Source: CAD feature listing. Evaluate the final solid. Frame: model axes, mm. A direction names the side the tool comes from. Give positions to 0.01 mm unless a question says otherwise; leave off trailing zeros. Write each loop counter-clockwise with the first axis right and the second up, starting at its lowest first coordinate (ties: lowest second). Pieces come first, ordered by that corner, then holes. Notation, with made-up numbers: M 71,87.5 L 120,87.5 A18 cw 120,95.5 Z; hole C 62.25,3 d9. An arc over 180 degrees is marked long. Use CSV: the item, a comma, the result in double quotes. Start each with the question number.
from build123d import *

# Parameters (mm, degrees)
F1_DEPTH = 240
F2_T     = -15
F3_R     = 50
F4_DEPTH = 50
F5_R     = 75
F6_DEPTH = 50


with BuildPart() as f1:
    # F0 (on Top) → F1 (new body)
    with BuildSketch(Plane.XY):
        with BuildLine():
            Line((0, 420), (0, 0))
            Line((0, 0), (300, 0))
            Line((300, 0), (300, 120))
            Line((300, 120), (220, 120))
            Line((220, 120), (220, 320))
            ThreePointArc((220, 320), (187.6502089709, 540.8304597359), (0, 420))
        make_face()
    extrude(amount=F1_DEPTH)

    # F2
    f2_openings = [f1.faces().sort_by_distance(p)[0] for p in [
        (150, 0, 120),
    ]]
    offset(amount=F2_T, openings=f2_openings, kind=Kind.INTERSECTION)

    # F3 (on face) → F4 (cut)
    with BuildSketch(Plane.XY.offset(240)):
        with Locations((132.7272727273, 420)):
            Circle(F3_R)
    extrude(amount=-F4_DEPTH, mode=Mode.SUBTRACT)

    # F5 (on face) → F6 (cut)
    with BuildSketch(Plane(origin=(0, 0, 0), x_dir=(0, -1, 0), z_dir=(-1, 0, 0))):
        with Locations((-320, 120)):
            Circle(F5_R)
        with Locations((-120, 120)):
            Circle(F5_R)
    extrude(amount=-F6_DEPTH, mode=Mode.SUBTRACT)


solid = f1.part
1. Access query for faces 5 (the cylindrical face through (7.395, 248.463, 142.528)), 6 (the cylindrical face through (126.218, 469.575, 232.605)), 7 (the flat face through (261, 120, 118)), 8 (the flat face through (0, 213, 118)), 9 (the flat face through (205, 214, 119)). Directions: +Z, -Z, +X, -X, +Y, -Y. A direction counts if a zero-diameter tool reaches every point of the face in a straight line with its end or side. Return the directions, or none.
2. Pull-direction query (Z, two-part tool) for faces 1 (the flat face through (300, 59, 118)), 2 (the cylindrical face through (187.432, 524.246, 118.53)), 3 (the flat face through (115, 280, 0)), 4 (the flat face through (115, 280, 240)); classes: released by +Z, released by -Z, zero draft, split by the parting line, or undercut.
3. Section A-A on z = 120. Return loops of the section in (x, y).
4. Section D-D on x = 74.5. Return loops of the section in (y, z), then the cut area to 3 significant figures.
5. Line query: probe 1 along Z at (x, y) = (32, 215.5); probe 2 along Z at (x, y) = (7, 320); probe 3 along X at (y, z) = (223, 199). Output: solid intervals per line, ascending.
6. First-contact query: pin 1 (1.5 mm diameter, centred on y = 442, z = 48.5, fed in from +X); pin 2 (10 mm diameter, centred on y = 282, z = 173.5, fed in from +X); pin 3 (6 mm diameter, centred on y = 437, z = 58.5, fed in from +X). Flat tips, straight axial feed; report the tip coordinate or a pass-through.
7. Section C-C on y = 389. Return loops of the section in (x, z), then the cut area to 3 significant figures.
8. Section B-B on y = 205. Return loops of the section in (x, z).
Resolved:
1,face 5,"-X"
1,face 6,"+Z"
1,face 7,"+Z, -Z, +X"
1,face 8,"+Z, -Z, -X, +Y, -Y"
1,face 9,"-Y"
2,face 1,"zero draft"
2,face 2,"undercut"
2,face 3,"released by -Z"
2,face 4,"released by +Z"
3,outline,"M 0,0 L 15,0 L 15,45 L 0,45 Z; M 0,195 L 15,195 L 15,245 L 0,245 Z; M 0,395 L 15,395 L 15,420 A117.73 cw long 205,327.07 L 205,105 L 285,105 L 285,0 L 300,0 L 300,120 L 220,120 L 220,320 A132.73 ccw long 0,420 Z"
4,outline,"M 0,0 L 539.27,0 L 539.27,240 L 0,240 L 0,225 L 522.32,225 L 522.32,15 L 0,15 Z"
4,area,"19,700 mm2"
5,probe 1,"z = 0 to 15, 225 to 240"
5,probe 2,"z = 0 to 45, 195 to 240"
5,probe 3,"x = 0 to 15, 205 to 220"
6,pin 1,"stops at x = 263.74"
6,pin 2,"stops at x = 220"
6,pin 3,"stops at x = 264.71"
7,outline,"M 0,0 L 261.78,0 L 261.78,240 L 171.96,240 L 171.96,225 L 246.3,225 L 246.3,15 L 15,15 L 15,90.61 L 0,90.61 Z; M 0,149.39 L 15,149.39 L 15,225 L 93.5,225 L 93.5,240 L 0,240 Z"
7,area,"12,200 mm2"
8,outline,"M 0,0 L 220,0 L 220,240 L 0,240 Z; hole M 15,15 L 205,15 L 205,225 L 15,225 Z"
